Verification items for the finished model (mm, model axes). A direction names the side the tool comes from. Give positions to 0.01 mm unless a question says otherwise; leave off trailing zeros. Write each loop counter-clockwise with the first axis right and the second up, starting at its lowest first coordinate (ties: lowest second). Pieces come first, ordered by that corner, then holes. Notation, with made-up numbers: (75, 54.5) -> (89, 54.5) arc R21 cw to (89, 92.5) -> close; hole circle Ø9 at (33.25, 30). An arc over 180 degrees is marked (long way). Write item = value, one per line.
from build123d import *

# Parameters (mm, degrees)
SKETCH1_W           = 27
SKETCH1_H           = 20
SKETCH1_R           = 1.2192
BOSS_EXTRUDE1_DEPTH = 1.524
SKETCH3_W           = 2.413
SKETCH3_H           = 2.413
BOSS_EXTRUDE2_DEPTH = 2.54
SKETCH4_W           = 0.635
SKETCH4_H           = 0.635
BOSS_EXTRUDE3_DEPTH = 5.715
FILLET1_R           = 2.54
SKETCH5_W           = 7.7851
SKETCH5_H           = 3.2512
SKETCH5_R           = 0.381
BOSS_EXTRUDE4_DEPTH = 2.1971


with BuildPart() as part:
    # Sketch1 → Boss-Extrude1 (new body)
    with BuildSketch(Plane(origin=(0, 0, 0), x_dir=(1, 0, 0), z_dir=(0, 1, 0))):
        with Locations((13.5, 10)):
            Rectangle(SKETCH1_W, SKETCH1_H)
        with Locations((2.5, 17.5)):
            Circle(SKETCH1_R, mode=Mode.SUBTRACT)
        with Locations((24.5, 17.5)):
            Circle(SKETCH1_R, mode=Mode.SUBTRACT)
        with Locations((24.5, 2.5)):
            Circle(SKETCH1_R, mode=Mode.SUBTRACT)
        with Locations((2.5, 2.5)):
            Circle(SKETCH1_R, mode=Mode.SUBTRACT)
    extrude(amount=BOSS_EXTRUDE1_DEPTH)

    # Sketch3 → Boss-Extrude2 (add)
    with BuildSketch(Plane(origin=(0, 0, 0), x_dir=(-1, 0, 0), z_dir=(0, -1, 0))):
        with Locations((-19.85, -0.9525)):
            Rectangle(SKETCH3_W, SKETCH3_H)
        with Locations((-14.77, -0.9525)):
            Rectangle(SKETCH3_W, SKETCH3_H)
        with Locations((-12.23, -0.9525)):
            Rectangle(SKETCH3_W, SKETCH3_H)
        with Locations((-9.69, -0.9525)):
            Rectangle(SKETCH3_W, SKETCH3_H)
        with Locations((-7.15, -0.9525)):
            Rectangle(SKETCH3_W, SKETCH3_H)
        with Locations((-17.31, -0.9525)):
            Rectangle(SKETCH3_W, SKETCH3_H)
    extrude(amount=BOSS_EXTRUDE2_DEPTH)

    # Sketch4 → Boss-Extrude3 (add)
    with BuildSketch(Plane.XY.offset(2.159)):
        with Locations((17.31, -1.27)):
            Rectangle(SKETCH4_W, SKETCH4_H)
        with Locations((7.15, -1.27)):
            Rectangle(SKETCH4_W, SKETCH4_H)
        with Locations((9.69, -1.27)):
            Rectangle(SKETCH4_W, SKETCH4_H)
        with Locations((12.23, -1.27)):
            Rectangle(SKETCH4_W, SKETCH4_H)
        with Locations((14.77, -1.27)):
            Rectangle(SKETCH4_W, SKETCH4_H)
        with Locations((19.85, -1.27)):
            Rectangle(SKETCH4_W, SKETCH4_H)
    extrude(amount=BOSS_EXTRUDE3_DEPTH)

    # Fillet1
    fillet1_edges = [part.edges().sort_by_distance(p)[0] for p in [
        (0, 0.762, -20),
        (27, 0.762, -20),
        (27, 0.762, 0),
        (0, 0.762, 0),
    ]]
    fillet(fillet1_edges, radius=FILLET1_R)

    # Sketch5 → Boss-Extrude4 (add)
    with BuildSketch(Plane.XZ):
        with Locations((21.287352133, -11.916943925)):
            Rectangle(SKETCH5_W, SKETCH5_H)
        with Locations((23.50781589, -11.916943925)):
            Circle(SKETCH5_R, mode=Mode.SUBTRACT)
    extrude(amount=BOSS_EXTRUDE4_DEPTH)


solid = part.part
Item 1: Mould release check, pull along Z, two halves, no side actions. Record for faces 1 (the flat face through (10, -1, -0.254)), 2 (the flat face through (10, 0, 1)), 3 (the flat face through (20, -1, -0.254)): +Z half, -Z half, draft (parallel to the pull), parting line (faces both ways), or undercut.
Response values:
face_1 = -Z half
face_2 = draft
face_3 = undercut
Item 2: Go/stop test with flat-tipped pins: P1, Ø0.7, axis at x = 17.5, z = 4.5, coming from the -Y side; P2, Ø0.5, axis at y = -1.5, z = 4, coming from the +X side; P3, Ø0.7, axis at x = 9.5, z = 4.5, coming from the +Y side; P4, Ø1.2, axis at x = 19.5, y = -1, coming from the +Z side. Record where each tip stops, or that it passes through.
Response values:
P1 = -1.59
P2 = 20.17
P3 = -0.95
P4 = 7.87
Item 3: Sectioned sample at B-B on x = 22.75. Record the cut outline in (y, z).
Response values:
outline = (-2.2, -13.54) -> (0, -13.54) -> (0, -20) -> (1.52, -20) -> (1.52, 0) -> (0, 0) -> (0, -10.29) -> (-2.2, -10.29) -> close
Item 4: Set-up check for faces 4 (the flat face through (20, 0, 1)), 5 (the flat face through (7, -2.54, 1)), 6 (the flat face through (17.395, -1, -12)): record each of +Z, -Z, +X, -X, +Y, -Y from which the full face is reachable in a straight line by a thin tool's end or side.
Response values:
face_4 = +Z, +X, -X, +Y
face_5 = +Z, -Z, +X, -X, -Y
face_6 = -Z, -X, -Y
Item 5: Sectioned sample at A-A on y = 0.85. Record the cut outline in (x, z), then the cut area to 3 significant figures.
Response values:
outline = (0, -17.46) arc R2.54 ccw to (2.54, -20) -> (24.46, -20) arc R2.54 ccw to (27, -17.46) -> (27, -2.54) arc R2.54 ccw to (24.46, 0) -> (2.54, 0) arc R2.54 ccw to (0, -2.54) -> close; hole circle Ø2.44 at (2.5, -17.5); hole circle Ø2.44 at (2.5, -2.5); hole circle Ø2.44 at (24.5, -17.5); hole circle Ø2.44 at (24.5, -2.5)
area = 516 mm^2
Item 6: Sectioned sample at D-D on x = 13. Record the cut outline in (y, z).
Response values:
outline = (-2.54, -0.25) -> (0, -0.25) -> (0, -20) -> (1.52, -20) -> (1.52, 0) -> (0, 0) -> (0, 2.16) -> (-2.54, 2.16) -> close
Item 7: Sectioned sample at C-C on z = -5. Record the cut outline in (x, y).
Response values:
outline = (0, 0) -> (27, 0) -> (27, 1.52) -> (0, 1.52) -> close
Item 8: Material ranges on line 1 (X direction, y = 0.9, z = -2.5); line 2 (Z direction, x = 24.5, y = 0.65); line 3 (X direction, y = 0.85, z = -18.25), recorded low to high.
Response values:
line_1 = 0 to 1.28, 3.72 to 23.28, 25.72 to 27
line_2 = -20 to -18.72, -16.28 to -3.72, -1.28 to 0
line_3 = 0.13 to 1.54, 3.46 to 23.54, 25.46 to 26.87
